Work out the finished part from the listing and answer in its coordinate system (mm). A direction names the side the tool comes from. Round coordinates to 2 decimals unless told otherwise and drop trailing zeros. Loops run counter-clockwise (first coordinate to the right, second up) from the corner with the lowest first, then second, coordinate; pieces in that order, holes last.
Autodesk Inventor part; units mm, degrees
ref_plane "作業平面1" through (0, -32.2, 0) normal (0, 1, 0) x (-1, 0, 0)
ref_plane "YZ Plane" through (0, 0, 0) normal (1, 0, 0) x (0, 1, 0)
ref_plane "XY Plane" through (0, 0, 0) normal (0, 0, 1) x (1, 0, 0)
sketch "スケッチ1" plane through (0, 0, 0) normal (1, 0, 0) x (0, 1, 0)
  line L0 (0, 41.3) -> (0, -41.3)
  line L1 (-39, 0) -> (17, 0)
  line L2 (-5.2, 19) -> (3.2, 19)
  line L3 (3.2, 19) -> (3.2, 17)
  line L4 (3.2, 17) -> (0, 17)
  line L5 (0, 17) -> (0, 9.3)
  line L6 (0, 9.3) -> (3.2, 9.3)
  line L7 (3.2, 9.3) -> (3.2, 6.9)
  line L8 (3.2, 6.9) -> (0, 6.9)
  line L9 (0, 6.9) -> (0, -6.9)
  line L10 (0, -6.9) -> (3.2, -6.9)
  line L11 (3.2, -6.9) -> (3.2, -9.3)
  line L12 (3.2, -9.3) -> (0, -9.3)
  line L13 (0, -9.3) -> (0, -17)
  line L14 (0, -17) -> (3.2, -17)
  line L15 (3.2, -17) -> (3.2, -19)
  line L16 (3.2, -19) -> (-5.2, -19)
  line L17 (-5.2, -19) -> (-5.2, 19)
  line L18 (-5.2, 27.5) -> (-5.2, -27.5)
  line L19 (-5.2, -27.5) -> (9, -27.5)
  line L20 (9, -27.5) -> (9, -29.5)
  line L21 (9, -29.5) -> (-11, -29.5)
  line L22 (-11, -29.5) -> (-11, 29.5)
  line L23 (-11, 29.5) -> (9, 29.5)
  line L24 (9, 29.5) -> (9, 27.5)
  line L25 (9, 27.5) -> (-5.2, 27.5)
  line L26 (-11, 29.5) -> (-22.3278, 16)
  line L27 (-22.3278, 16) -> (-31, 16)
  line L28 (-31, 16) -> (-31, 12)
  line L29 (-31, 12) -> (-21.0692, 12)
  line L30 (-21.0692, 12) -> (-11, 0)
  line L31 (-11, 0) -> (-21.0692, -12)
  line L32 (-21.0692, -12) -> (-31, -12)
  line L33 (-31, -12) -> (-31, -16)
  line L34 (-31, -16) -> (-22.3278, -16)
  line L35 (-22.3278, -16) -> (-11, -29.5)
  point P0 (0, 0)
  dimension "d0" = 38
  dimension "d1" = 18.6
  dimension "d2" = 2
  dimension "d3" = 2.4
  dimension "d4" = 3.2
  dimension "d5" = 8.4
  dimension "d6" = 59
  dimension "d7" = 2
  dimension "d8" = 20
  dimension "d9" = 5.8
  dimension "d10" = 5.8
  dimension "d11" = 40
  dimension "d12" = 40
  dimension "d13" = 32
  dimension "d14" = 4
  dimension "d15" = 20
extrude "押し出し1" add sketch "スケッチ1" along normal mid plane 23.75 contours L0 L1 L17 L2 | L0 L2 L3 L4 | L6 L7 L8 L0 | L0 L16 L17 L1 | L10 L11 L12 L0 | L0 L14 L15 L16
extrude "押し出し2" add sketch "スケッチ1" along normal mid plane 83.75 contours L25 L18 L17 L1 L22 L23 L0 | L0 L23 L24 L25 | L17 L18 L19 L0 L21 L22 L1 | L22 L30 L29 L28 L27 L26 | L22 L35 L34 L33 L32 L31 | L0 L19 L20 L21
ref_plane "作業平面1" through (0, -32.2, 0) normal (0, 1, 0) x (-1, 0, 0)
sketch "スケッチ2" plane through (0, -32.2, 0) normal (0, 1, 0) x (-1, 0, 0)
  line L0 (0, -41.3) -> (0, 41.3)
  line L1 (-58.625, 0) -> (58.625, 0)
  line L2 (31.875, -19) -> (21.875, -19)
  line L3 (21.875, -19) -> (21.875, -9)
  line L4 (21.875, -9) -> (31.875, -9)
  line L5 (31.875, -9) -> (31.875, -19)
  line L6 (-21.875, -19) -> (-31.875, -19)
  line L7 (-31.875, -19) -> (-31.875, -9)
  line L8 (-31.875, -9) -> (-21.875, -9)
  line L9 (-21.875, -9) -> (-21.875, -19)
  line L10 (31.875, 9) -> (21.875, 9)
  line L11 (21.875, 9) -> (21.875, 19)
  line L12 (21.875, 19) -> (31.875, 19)
  line L13 (31.875, 19) -> (31.875, 9)
  line L14 (-21.875, 9) -> (-31.875, 9)
  line L15 (-31.875, 9) -> (-31.875, 19)
  line L16 (-31.875, 19) -> (-21.875, 19)
  line L17 (-21.875, 19) -> (-21.875, 9)
  line L18 (-21.875, 16.2551) -> (21.875, 16.2551)
  line L19 (21.875, 16.2551) -> (21.875, 12)
  line L20 (21.875, 12) -> (-21.875, 12)
  line L21 (-21.875, 12) -> (-21.875, 16.2551)
  line L22 (21.875, -12) -> (-21.875, -12)
  line L23 (-21.875, -12) -> (-21.875, -16.2551)
  line L24 (-21.875, -16.2551) -> (21.875, -16.2551)
  line L25 (21.875, -16.2551) -> (21.875, -12)
  line L26 (-28.875, 9) -> (-24.875, 9)
  line L27 (-24.875, 9) -> (-24.875, -9)
  line L28 (-24.875, -9) -> (-28.875, -9)
  line L29 (-28.875, -9) -> (-28.875, 9)
  line L30 (24.875, 9) -> (28.875, 9)
  line L31 (28.875, 9) -> (28.875, -9)
  line L32 (28.875, -9) -> (24.875, -9)
  line L33 (24.875, -9) -> (24.875, 9)
  point P0 (0, 0)
  dimension "d21" = 38
  dimension "d23" = 53.75
  dimension "d24" = 10
  dimension "d25" = 10
  dimension "d28" = 3
  dimension "d29" = 3
  dimension "d30" = 3
  dimension "d31" = 2.7449
extrude "押し出し3" add sketch "スケッチ2" along normal up to next contours L24 L9 L22 L0 | L0 L22 L3 L24 | L9 L6 L7 L8 | L3 L4 L5 L2 | L20 L17 L18 L0 | L0 L18 L11 L20 | L27 L8 L29 L1 | L1 L29 L14 L27 | L33 L10 L31 L1 | L1 L31 L4 L33 | L11 L12 L13 L10 | L17 L14 L15 L16
sketch "スケッチ3" plane through (0, 0, 0) normal (0, 0, 1) x (1, 0, 0)
  line L0 (-41.875, -11) -> (-31.875, -31)
  line L1 (-31.875, -31) -> (-41.875, -31)
  line L2 (-41.875, -31) -> (-41.875, -11)
  line L3 (0, 17.24) -> (0, -40.44)
  line L4 (41.875, -11) -> (31.875, -31)
  line L5 (31.875, -31) -> (41.875, -31)
  line L6 (41.875, -31) -> (41.875, -11)
  point P0 (0, 0)
extrude "押し出し4" cut sketch "スケッチ3" against normal through all both and the other way through all
equation "\"d0\" = RailWidth"
equation "\"d1\" = InsideWidth"
equation "\"d2\" = OuterWall"
equation "\"d3\" = InnerWall"
equation "\"d4\" = RailDepth"
equation "\"d5\" = RailHeight"
equation "\"d9\" = d10"
equation "\"d16\" = Length - 2 * ConnectorLength"
equation "\"d21\" = RailWidth"
equation "\"d23\" = Length"
equation "\"d29\" = d28"
equation "\"d30\" = d28"
equation "\"Length\" = 0.25 * StraightLength"
properties part number "Viaduct_HorizontalSingle"
Item 1: Determine the mould class of faces 1 (the face through (0, 3.2, -18)), 2 (the face through (11.875, -2, 0)), 3 (the face through (-23, -25, 9)) for opening direction X: pulls with the +X half, pulls with the -X half, needs draft (parallel to the pull), parting line crosses it, or undercut.
Item 2: Section D-D, the plane z = -10.5 is taken. Give the vertices of the cut face in (x, y) (3 decimals), plus the area to 3 significant figures.
Item 3: For faces 4 (the face through (-21.875, -25, 10)), 5 (the face through (-1, 2, 27.5)), 6 (the face through (-27, -26, -19)), determine the directions among +Z, -Z, +X, -X, +Y, -Y from which every point of the face is accessible in a straight line to the end or side of a thin tool.
Item 4: Section A-A, the plane x = -23.5 is taken. Give the vertices of the cut face in (y, z), plus the area to 3 significant figures.
Item 5: Section B-B, the plane z = -1 is taken. Give the vertices of the cut face in (x, y) (3 decimals), plus the area to 3 significant figures.
Item 6: Each of these flat-tipped pins is pushed along its axis until it touches: P1, Ø0.9, axis at y = -26.5, z = -11, coming from the -X side (3 decimals); P2, Ø12, axis at x = -4, y = -25.5, coming from the +Z side; P3, Ø1.5, axis at x = 6, z = -0.5, coming from the -Y side. Where does it stop, or does it pass through?
Item 7: Section C-C, the plane x = 13.5 is taken. Give the vertices of the cut face in (y, z), plus the area to 3 significant figures.
Item 8: Straight lines are drawn through the part: line 1 (Z direction, x = 1, y = 7); line 2 (Z direction, x = -31, y = -29); line 3 (X direction, y = -24, z = 7) (3 decimals). For each, find the intervals that lie inside material, in ascending order.
Answer below:
1. face 1: needs draft
1. face 2: pulls with the +X half
1. face 3: undercut
2. outline: (-41.875, -11) - (-37.47, -19.811) - (-31.875, -19.811) - (-31.875, -32.2) - (-21.875, -32.2) - (-21.875, -19.811) - (21.875, -19.811) - (21.875, -32.2) - (31.875, -32.2) - (31.875, -19.811) - (37.47, -19.811) - (41.875, -11) - (41.875, -5.2) - (11.875, -5.2) - (11.875, 0) - (-11.875, 0) - (-11.875, -5.2) - (-41.875, -5.2) - close
2. area: 1,560 mm2
3. face 4: -Y
3. face 5: +X, -X, +Y
3. face 6: -Z, +X, -X, -Y
4. outline: (-32.2, -19) - (-19.81, -19) - (-11, -29.5) - (9, -29.5) - (9, -27.5) - (-5.2, -27.5) - (-5.2, 27.5) - (9, 27.5) - (9, 29.5) - (-11, 29.5) - (-19.81, 19) - (-32.2, 19) - (-32.2, 9) - (-18.55, 9) - (-11, 0) - (-18.55, -9) - (-32.2, -9) - close
4. area: 983 mm2
5. outline: (-41.875, -11) - (-41.455, -11.839) - (-28.875, -11.839) - (-28.875, -32.2) - (-24.875, -32.2) - (-24.875, -11.839) - (24.875, -11.839) - (24.875, -32.2) - (28.875, -32.2) - (28.875, -11.839) - (41.455, -11.839) - (41.875, -11) - (41.875, -5.2) - (11.875, -5.2) - (11.875, 0) - (-11.875, 0) - (-11.875, -5.2) - (-41.875, -5.2) - close
5. area: 842 mm2
6. P1: stops at x = -31.875
6. P2: stops at z = 19.37
6. P3: stops at y = -12.05
7. outline: (-32.2, -16.26) - (-22.11, -16.26) - (-11, -29.5) - (9, -29.5) - (9, -27.5) - (-5.2, -27.5) - (-5.2, 27.5) - (9, 27.5) - (9, 29.5) - (-11, 29.5) - (-22.11, 16.26) - (-32.2, 16.26) - (-32.2, 12) - (-21.07, 12) - (-11, 0) - (-21.07, -12) - (-32.2, -12) - close
7. area: 847 mm2
8. line 1: z = -29.5 to -27.5, 27.5 to 29.5
8. line 2: z = -19 to -9, 9 to 19
8. line 3: x = -28.875 to -24.875, 24.875 to 28.875
